Geometry check sheet. Reference: the model listing, model coordinates, mm. A direction names the side the tool comes from. Round coordinates to 2 decimals unless told otherwise and drop trailing zeros. Write each loop counter-clockwise with the first axis right and the second up, starting at its lowest first coordinate (ties: lowest second). Pieces come first, ordered by that corner, then holes. Notation, with made-up numbers: M 47.25,-8 L 84.25,-8 A14 ccw 84.25,-4 Z; hole C 6.25,69 d5. An arc over 180 degrees is marked long. Use a Markdown table: item, result.
```python
from build123d import *

# Parameters (mm, degrees)
SKETCH1_W           = 92.6
SKETCH1_H           = 300
BOSS_EXTRUDE1_DEPTH = 2
SKETCH2_R           = 2.25
SKETCH2_W           = 8.48
SKETCH2_H           = 51.5
SKETCH2_H_2         = 50
SKETCH2_H_3         = 53
CUT_EXTRUDE1_DEPTH  = 10
FILLET1_R           = 2
CUT_EXTRUDE3_DEPTH  = 8.5
SKETCH5_R           = 1.85
CUT_EXTRUDE4_DEPTH  = 10


with BuildPart() as part:
    # Sketch1 → Boss-Extrude1 (new body)
    with BuildSketch(Plane.XY):
        Rectangle(SKETCH1_W, SKETCH1_H)
    extrude(amount=BOSS_EXTRUDE1_DEPTH)

    # Sketch2 → Cut-Extrude1 (cut)
    with BuildSketch(Plane.XY):
        with Locations((-42.06, 75)):
            Circle(SKETCH2_R)
        with Locations((42.06, 125)):
            Circle(SKETCH2_R)
        with Locations((42.06, 25)):
            Circle(SKETCH2_R)
        with Locations((42.06, -75)):
            Circle(SKETCH2_R)
        with Locations((-42.06, -25)):
            Circle(SKETCH2_R)
        with Locations((-42.06, -125)):
            Circle(SKETCH2_R)
        with Locations((-42.06, 124.25)):
            Rectangle(SKETCH2_W, SKETCH2_H)
        with Locations((42.06, 75)):
            Rectangle(SKETCH2_W, SKETCH2_H_2)
        with Locations((42.06, -25)):
            Rectangle(SKETCH2_W, SKETCH2_H_2)
        with Locations((-42.06, 25)):
            Rectangle(SKETCH2_W, SKETCH2_H_3)
        with Locations((-42.06, -75)):
            Rectangle(SKETCH2_W, SKETCH2_H_3)
        with Locations((42.06, -125)):
            Rectangle(SKETCH2_W, SKETCH2_H_2)
    extrude(amount=CUT_EXTRUDE1_DEPTH, mode=Mode.SUBTRACT)

    # Fillet1
    fillet1_edges = [part.edges().sort_by_distance(p)[0] for p in [
        (46.3, -100, 1),
        (37.82, -100, 1),
        (37.82, -150, 1),
        (46.3, 50, 1),
        (46.3, 100, 1),
        (37.82, 100, 1),
        (37.82, 50, 1),
        (-46.3, -48.5, 1),
        (-46.3, -101.5, 1),
        (-37.82, -101.5, 1),
        (-37.82, -48.5, 1),
        (37.82, 0, 1),
        (37.82, -50, 1),
        (46.3, -50, 1),
        (46.3, 0, 1),
        (46.3, 150, 1),
        (-46.3, -150, 1),
        (-46.3, 51.5, 1),
        (-46.3, -1.5, 1),
        (-37.82, -1.5, 1),
        (-37.82, 51.5, 1),
        (-46.3, 98.5, 1),
        (-37.82, 98.5, 1),
        (-37.82, 150, 1),
    ]]
    fillet(fillet1_edges, radius=FILLET1_R)

    # Sketch4 → Cut-Extrude3 (cut)
    with BuildSketch(Plane(origin=(0, 0, 0), x_dir=(-1, 0, 0), z_dir=(0, 0, -1))):
        with BuildLine():
            Line((25, 93), (-25, 93))
            ThreePointArc((-25, 93), (-28.535533906, 94.464466094), (-30, 98))
            Line((-30, 98), (-30, 138))
            ThreePointArc((-30, 138), (-28.535533906, 141.535533906), (-25, 143))
            Line((-25, 143), (25, 143))
            ThreePointArc((25, 143), (28.535533906, 141.535533906), (30, 138))
            Line((30, 138), (30, 98))
            ThreePointArc((30, 98), (28.535533906, 94.464466094), (25, 93))
        make_face()
        with BuildLine():
            Line((25, -143), (-25, -143))
            ThreePointArc((-25, -143), (-28.535533906, -141.535533906), (-30, -138))
            Line((-30, -138), (-30, -98))
            ThreePointArc((-30, -98), (-28.535533906, -94.464466094), (-25, -93))
            Line((-25, -93), (25, -93))
            ThreePointArc((25, -93), (28.535533906, -94.464466094), (30, -98))
            Line((30, -98), (30, -138))
            ThreePointArc((30, -138), (28.535533906, -141.535533906), (25, -143))
        make_face()
    extrude(amount=-CUT_EXTRUDE3_DEPTH, mode=Mode.SUBTRACT)

    # Sketch5 → Cut-Extrude4 (cut)
    with BuildSketch(Plane(origin=(0, 0, 0), x_dir=(-1, 0, 0), z_dir=(0, 0, -1))):
        with Locations((-16.43, 46)):
            Circle(SKETCH5_R)
        with Locations((-0.18, 76.2)):
            Circle(SKETCH5_R)
    extrude(amount=-CUT_EXTRUDE4_DEPTH, mode=Mode.SUBTRACT)


solid = part.part
```
Item 1: Access from +Z, -Z, +X, -X, +Y, -Y to the whole of each face (thin tool, end or side, straight path). Record for faces 1 (the face through (-1, 2, 2)), 2 (the face through (28, -142, 1)).
Outcome:
| item | result |
|---|---|
| face 1 | +Z, +X, -X, +Y, -Y |
| face 2 | +Z, -Z |
Item 2: Mould release check, pull along X, two halves, no side actions. Record for faces 3 (the face through (29, 141, 1)), 4 (the face through (-1, 2, 0)): +X half, -X half, draft (parallel to the pull), parting line (faces both ways), or undercut.
Outcome:
| item | result |
|---|---|
| face 3 | undercut |
| face 4 | draft |
Item 3: Material ranges on line 1 along Y through (x, z) = (0.18, 1.15); line 2 along Y through (x, z) = (42.06, 1.25); line 3 along Y through (x, z) = (16.43, 1.3), recorded low to high. Write a range as from..to.
Outcome:
| item | result |
|---|---|
| line 1 | y = -150..-143, -93..74.35, 78.05..93, 143..150 |
| line 2 | y = -100..-77.25, -72.75..-50, 0..22.75, 27.25..50, 100..122.75, 127.25..150 |
| line 3 | y = -150..-143, -93..44.15, 47.85..93, 143..150 |
Item 4: Cross-section at A-A, the plane x = -18. Record the cut outline in (y, z).
Outcome:
| item | result |
|---|---|
| outline | M -150,0 L -143,0 L -143,2 L -150,2 Z; M -93,0 L 93,0 L 93,2 L -93,2 Z; M 143,0 L 150,0 L 150,2 L 143,2 Z |
Item 5: Go/stop test with flat-tipped pins: pin 1 (7 mm diameter, centred on x = 42.06, y = -75, fed in from -Z); pin 2 (1 mm diameter, centred on y = 119, z = 1, fed in from -X); pin 3 (1 mm diameter, centred on x = -41.5, z = 1, fed in from +Y). Record where each tip stops, or that it passes through.
Outcome:
| item | result |
|---|---|
| pin 1 | stops at z = 0 |
| pin 2 | stops at x = -37.82 |
| pin 3 | stops at y = 98.5 |
Item 6: Cross-section at B-B, the plane y = -120. Record the cut outline in (x, z), and give its area (3 significant figures).
Outcome:
| item | result |
|---|---|
| outline | M -46.3,0 L -30,0 L -30,2 L -46.3,2 Z; M 30,0 L 37.82,0 L 37.82,2 L 30,2 Z |
| area | 48.2 mm2 |
Item 7: Cross-section at D-D, the plane y = 83. Record the cut outline in (x, z).
Outcome:
| item | result |
|---|---|
| outline | M -46.3,0 L 37.82,0 L 37.82,2 L -46.3,2 Z |
Item 8: Cross-section at C-C, the plane z = 0.4. Count the separate pieces of the cut face and the enclosed holes in it, and give its area (3 significant figures).
Outcome:
| item | result |
|---|---|
| separate pieces | 1 |
| enclosed holes | 10 |
| area | 19,100 mm2 |
